from build123d import *

# Parameters (mm, degrees)
F0_R     = 3.25
F1_DEPTH = 13
F0_R_2   = 1
F2_DEPTH = 14
F3_DEPTH = 24
F4_DEPTH = 3
F5_R     = 1
F6_SIZE  = 1.25


with BuildPart() as f1:
    # F0 (on Top) → F1 (new body)
    with BuildSketch(Plane.XY):
        with BuildLine():
            ThreePointArc((12.085632, -2), (12.208839, -1.003371), (12.25, 0))
            ThreePointArc((12.25, 0), (12.208839, 1.003371), (12.085632, 2))
            ThreePointArc((12.085632, 2), (-12.25, 0), (12.085632, -2))
        make_face()
        Circle(F0_R, mode=Mode.SUBTRACT)
    extrude(amount=F1_DEPTH)

    # F0 (on Top) → F2 (join)
    with BuildSketch(Plane.XY):
        Circle(F0_R)
        Circle(F0_R_2, mode=Mode.SUBTRACT)
    extrude(amount=F2_DEPTH)

    # F0 (on Top) → F3 (join)
    with BuildSketch(Plane.XY):
        Circle(F0_R_2)
    extrude(amount=F3_DEPTH)

    # F0 (on Top) → F4 (join)
    with BuildSketch(Plane.XY):
        with BuildLine():
            ThreePointArc((12.085632, 2), (12.208839, 1.003371), (12.25, 0))
            ThreePointArc((12.25, 0), (12.208839, -1.003371), (12.085632, -2))
            Line((12.085632, -2), (14.085632, -2))
            Line((14.085632, -2), (14.085632, 2))
            Line((14.085632, 2), (12.085632, 2))
        make_face()
    extrude(amount=F4_DEPTH)

    # F5
    f5_edges = [f1.edges().sort_by_distance(p)[0] for p in [
        (-12.085632, 2, 13),
    ]]
    fillet(f5_edges, radius=F5_R)

    # F6
    f6_edges = [f1.edges().sort_by_distance(p)[0] for p in [
        (14.085632, -2, 1.5),
        (14.085632, 2, 1.5),
        (14.085632, 0, 0),
        (14.085632, 0, 3),
    ]]
    chamfer(f6_edges, length=F6_SIZE)


solid = f1.part
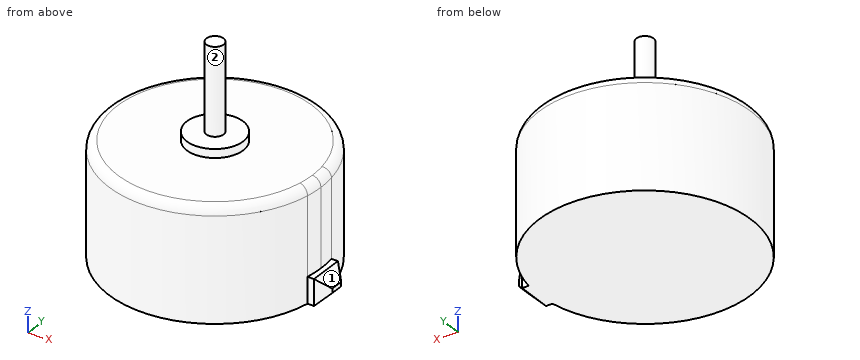
Could you check a few things on this model? Use its own coordinates, in mm. Face numbers are marked on the shaded views. A direction names the side the tool comes from. Coordinates: 2 decimals unless noted, no trailing zeros. Order: outer loops, then holes, each group sorted by start corner. A loop starts at its lowest first (then second) coordinate and runs counter-clockwise, first axis right, second up.
Q1. Suppose I cut it at B-B on z = 22.5. Please give me the cut outline in (x, y), and give its area (3 significant figures).
Q2. Will these pins go through, and if not, where does the flat tip stop? pin 1 (1 mm diameter, centred on y = 3, z = 20, fed in from -X); pin 2 (5 mm diameter, centred on x = 4.5, y = 8.5, fed in from +Z); pin 3 (6 mm diameter, centred on y = 1.5, z = 20, fed in from +X); pin 4 (5 mm diameter, centred on y = 5.5, z = 3, fed in from +X).
Q3. Suppose I cut it at A-A on z = 4.25. Please give me the cut outline in (x, y).
Q4. Which directions (+Z, -Z, +X, -X, +Y, -Y) give clear straight access to the entire face, cutting with the end or side of a thin tool? Please do the marked faces 1 and 2.
Q5. Please list where these lines run through material, in increasing order: L1, parallel to Z at x = -9.75, y = -4.75; L2, parallel to X at y = 0, z = 3.5; L3, parallel to Y at x = -7, z = 8.
Answer:
1. outline: circle Ø2 at (0, 0)
1. area: 3.14 mm2
2. pin 1: passes through
2. pin 2: stops at z = 13
2. pin 3: stops at x = 1
2. pin 4: stops at x = 11.88
3. outline: (12.09, -2) arc R12.25 ccw to (12.25, 0) arc R12.25 ccw to (12.09, 2) arc R12.25 ccw (long way) to start
4. face 1: +Z, +X, +Y, -Y
4. face 2: +Z
5. L1: z = 0 to 13
5. L2: x = -12.25 to 12.25
5. L3: y = -10.05 to 10.05
